Could you check a few things on this model? Use its own coordinates, in mm. Face numbers are marked on the shaded views. A direction names the side the tool comes from. Round coordinates to 2 decimals unless told otherwise and drop trailing zeros. Loops run counter-clockwise (first coordinate to the right, second up) from the corner with the lowest first, then second, coordinate; pieces in that order, holes last. Notation, with made-up numbers: M 66.25,39 L 73.25,39 A24 cw 73.25,70 Z; hole C 42,40.5 d2. An arc over 180 degrees is marked long. One line per item, written item: value. Start each with the question number.
Q1. Imagine slicing it at B-B (y = -62). Please give me the cut outline in (x, z).
Q2. Imagine slicing it at C-C (z = 29.95). Give the number of separate pieces and of enclosed holes in the cut face, then the cut area to 3 significant figures.
Q3. Which directions (+Z, -Z, +X, -X, +Y, -Y) give clear straight access to the entire face, cutting with the end or side of a thin tool? Please do the marked faces 4 and 5.
Q4. Imagine slicing it at A-A (z = 40). Please give me the cut outline in (x, y), then the cut area to 3 significant figures.
Q5. Thinking about a two-plate mould opening in Y: for the marked faces 1, 2 and 3, which applies, released by +Y, released by -Y, zero draft, split by the parting line, or undercut?
Q6. Please list where these lines run through material, in increasing order: line 1 along Y through (x, z) = (24.5, 20); line 2 along X through (y, z) = (-129, 64); line 3 along X through (y, z) = (7, 49.95).
Q7. Imagine slicing it at D-D (y = -124.5). Please give me the cut outline in (x, z), then the cut area to 3 significant figures.
Q8. I'm going to push flat-ended pins straight in: pin 1 Ø5.5 at (x, y) = (-38, -3) entering from -Z; pin 2 Ø10 at (x, y) = (19, -9.5) entering from +Z; pin 3 Ø9 at (x, y) = (-12, -93) entering from +Z. Where does each tip first touch, or does it pass through?
from build123d import *

# Parameters (mm, degrees)
SKETCH_1_W               = 160
SKETCH_1_H               = 170
EXTRUDE_1_DEPTH          = 3
SKETCH_9_W               = 160
SKETCH_9_H               = 170
SKETCH_9_W_2             = 154
SKETCH_9_H_2             = 164
EXTRUDE_6_DEPTH          = 75
SKETCH_10_R              = 4
SKETCH_10_R_2            = 1.55
EXTRUDE_7_DEPTH          = 20
SKETCH_11_W              = 14
SKETCH_11_H              = 14
CUT_EXTRUDE_3_DEPTH      = 20
SKETCH_12_R              = 22.5
CUT_EXTRUDE_4_DEPTH      = 10
SKETCH_13_W              = 15
SKETCH_13_H              = 35
CUT_EXTRUDE_5_DEPTH      = 10
SKETCH_14_W              = 10
SKETCH_14_H              = 10
EXTRUDE_8_DEPTH          = 10
SKETCH_15_W              = 4
SKETCH_15_H              = 7
CUT_EXTRUDE_6_DEPTH      = 10
SKETCH_16_R              = 1.6
CUT_EXTRUDE_7_DEPTH      = 20
MIRROR_4_COPY_1_SKETCH_W = 10
MIRROR_4_COPY_1_SKETCH_H = 10
MIRROR_4_COPY_1_DEPTH    = 10
MIRROR_4_COPY_2_SKETCH_W = 4
MIRROR_4_COPY_2_SKETCH_H = 7
MIRROR_4_COPY_2_DEPTH    = 10
MIRROR_4_COPY_3_SKETCH_R = 1.6
MIRROR_4_COPY_3_DEPTH    = 20
SKETCH_17_W              = 60
SKETCH_17_H              = 20
EXTRUDE_9_DEPTH          = 20
SKETCH_18_W              = 15
SKETCH_18_H              = 15
CUT_EXTRUDE_8_DEPTH      = 15
SKETCH_19_R              = 2.5
CUT_EXTRUDE_9_DEPTH      = 15
CUT_EXTRUDE_10_DEPTH     = 65


with BuildPart() as part:
    # 草图1 → 凸台-拉伸1 (new body)
    with BuildSketch(Plane.XY):
        with Locations((52.885281107, -76.271289123)):
            Rectangle(SKETCH_1_W, SKETCH_1_H)
    extrude(amount=EXTRUDE_1_DEPTH)

    # 草图9 → 凸台-拉伸6 (add)
    with BuildSketch(Plane.XY.offset(3)):
        with Locations((52.885281107, -76.271289123)):
            Rectangle(SKETCH_9_W, SKETCH_9_H)
        with Locations((52.885281107, -76.271289123)):
            Rectangle(SKETCH_9_W_2, SKETCH_9_H_2, mode=Mode.SUBTRACT)
    extrude(amount=EXTRUDE_6_DEPTH)

    # 草图10 → 凸台-拉伸7 (add)
    # profile 1 of 4: a face of its own
    with BuildSketch(Plane.XY.offset(3)):
        with Locations((-12.114718893, -0.271289123)):
            Circle(SKETCH_10_R)
        with Locations((-12.114718893, -0.271289123)):
            Circle(SKETCH_10_R_2, mode=Mode.SUBTRACT)
    # profile 2 of 4: a face of its own
    with BuildSketch(Plane.XY.offset(3)):
        with Locations((81.885281107, -0.271289123)):
            Circle(SKETCH_10_R)
        with Locations((81.885281107, -0.271289123)):
            Circle(SKETCH_10_R_2, mode=Mode.SUBTRACT)
    # profile 3 of 4: a face of its own
    with BuildSketch(Plane.XY.offset(3)):
        with Locations((-12.114718893, -94.271289123)):
            Circle(SKETCH_10_R)
        with Locations((-12.114718893, -94.271289123)):
            Circle(SKETCH_10_R_2, mode=Mode.SUBTRACT)
    # profile 4 of 4: a face of its own
    with BuildSketch(Plane.XY.offset(3)):
        with Locations((81.885281107, -94.271289123)):
            Circle(SKETCH_10_R)
        with Locations((81.885281107, -94.271289123)):
            Circle(SKETCH_10_R_2, mode=Mode.SUBTRACT)
    extrude(amount=EXTRUDE_7_DEPTH)

    # 草图11 → 切除-拉伸3 (cut)
    with BuildSketch(Plane(origin=(-24.114718893, 0, 0), x_dir=(0, 0, -1), z_dir=(1, 0, 0))):
        with Locations((-30.5, -83.221289123)):
            Rectangle(SKETCH_11_W, SKETCH_11_H)
    extrude(amount=-CUT_EXTRUDE_3_DEPTH, mode=Mode.SUBTRACT)

    # 草图12 → 切除-拉伸4 (cut)
    with BuildSketch(Plane.ZY.offset(27.114718893)):
        with Locations(Location((40, -126.271289123, 0), (0, 0, 270))):
            Circle(SKETCH_12_R)
    extrude(amount=-CUT_EXTRUDE_4_DEPTH, mode=Mode.SUBTRACT)

    # 草图13 → 切除-拉伸5 (cut)
    with BuildSketch(Plane.ZY.offset(27.114718893)):
        with Locations((55.5, -38.771289123)):
            Rectangle(SKETCH_13_W, SKETCH_13_H)
    extrude(amount=-CUT_EXTRUDE_5_DEPTH, mode=Mode.SUBTRACT)

    # 草图14 → 凸台-拉伸8 (add)
    with BuildSketch(Plane.XZ.offset(-5.728710877)):
        with Locations((-19.114718893, 73)):
            Rectangle(SKETCH_14_W, SKETCH_14_H)
    extrude_8 = extrude(amount=EXTRUDE_8_DEPTH)

    # 草图15 → 切除-拉伸6 (cut)
    with BuildSketch(Plane(origin=(-14.114718893, 0, 0), x_dir=(0, 0, -1), z_dir=(1, 0, 0))):
        with Locations((-72, 0.728710877)):
            Rectangle(SKETCH_15_W, SKETCH_15_H)
    cut_extrude_6 = extrude(amount=-CUT_EXTRUDE_6_DEPTH, mode=Mode.SUBTRACT)

    # 草图16 → 切除-拉伸7 (cut)
    with BuildSketch(Plane.XY.offset(78)):
        with Locations((-19.114718893, 0.728710877)):
            Circle(SKETCH_16_R)
    cut_extrude_7 = extrude(amount=-CUT_EXTRUDE_7_DEPTH, mode=Mode.SUBTRACT)

    # 镜向3: 凸台-拉伸8, 切除-拉伸6, 切除-拉伸7 across plane
    add(extrude_8.mirror(Plane.ZY.offset(-52.885281107)))
    add(cut_extrude_6.mirror(Plane.ZY.offset(-52.885281107)), mode=Mode.SUBTRACT)
    add(cut_extrude_7.mirror(Plane.ZY.offset(-52.885281107)), mode=Mode.SUBTRACT)

    # 镜向4: 凸台-拉伸8, 切除-拉伸6, 切除-拉伸7 across plane
    add(extrude_8.mirror(Plane.ZX.offset(-76.271289123)))
    add(cut_extrude_6.mirror(Plane.ZX.offset(-76.271289123)), mode=Mode.SUBTRACT)
    add(cut_extrude_7.mirror(Plane.ZX.offset(-76.271289123)), mode=Mode.SUBTRACT)

    # 镜向4 copy 1 sketch → 镜向4 copy 1 (add)
    with BuildSketch(Plane(origin=(105.770562214, -158.271289123, 0), x_dir=(-1, 0, 0), z_dir=(0, 1, 0))):
        with Locations((-19.114718893, 73)):
            Rectangle(MIRROR_4_COPY_1_SKETCH_W, MIRROR_4_COPY_1_SKETCH_H)
    extrude(amount=MIRROR_4_COPY_1_DEPTH)

    # 镜向4 copy 2 sketch → 镜向4 copy 2 (cut)
    with BuildSketch(Plane(origin=(119.885281107, -152.542578247, 0), x_dir=(0, 0, -1), z_dir=(-1, 0, 0))):
        with Locations((-72, 0.728710877)):
            Rectangle(MIRROR_4_COPY_2_SKETCH_W, MIRROR_4_COPY_2_SKETCH_H)
    extrude(amount=-MIRROR_4_COPY_2_DEPTH, mode=Mode.SUBTRACT)

    # 镜向4 copy 3 sketch → 镜向4 copy 3 (cut)
    with BuildSketch(Plane(origin=(105.770562214, -152.542578247, 78), x_dir=(-1, 0, 0), z_dir=(0, 0, 1))):
        with Locations((-19.114718893, 0.728710877)):
            Circle(MIRROR_4_COPY_3_SKETCH_R)
    extrude(amount=-MIRROR_4_COPY_3_DEPTH, mode=Mode.SUBTRACT)

    # 草图17 → 凸台-拉伸9 (add)
    with BuildSketch(Plane.ZY.offset(27.114718893)):
        with Locations((39, -1.271289123)):
            Rectangle(SKETCH_17_W, SKETCH_17_H)
    extrude_9 = extrude(amount=EXTRUDE_9_DEPTH)

    # 草图18 → 切除-拉伸8 (cut)
    with BuildSketch(Plane.ZY.offset(47.114718893)):
        with Locations((29.95, -3.771289123)):
            Rectangle(SKETCH_18_W, SKETCH_18_H)
        with Locations((49.95, -3.771289123)):
            Rectangle(SKETCH_18_W, SKETCH_18_H)
    cut_extrude_8 = extrude(amount=-CUT_EXTRUDE_8_DEPTH, mode=Mode.SUBTRACT)

    # 草图19 → 切除-拉伸9 (cut)
    with BuildSketch(Plane(origin=(0, 3.728710877, 0), x_dir=(-1, 0, 0), z_dir=(0, -1, 0))):
        with Locations(Location((39.614718893, -49.95, 0), (0, 0, 90))):
            Circle(SKETCH_19_R)
        with Locations(Location((39.614718893, -29.95, 0), (0, 0, 90))):
            Circle(SKETCH_19_R)
    cut_extrude_9 = extrude(amount=-CUT_EXTRUDE_9_DEPTH, mode=Mode.SUBTRACT)

    # 草图20 → 切除-拉伸10 (cut)
    with BuildSketch(Plane.XY.offset(69)):
        Polygon((-47.114718893, -11.271289123), (-27.114718893, -11.271289123), (-47.114718893, 5.558007734), align=None)
    cut_extrude_10 = extrude(amount=-CUT_EXTRUDE_10_DEPTH, mode=Mode.SUBTRACT)

    # 镜向5: 凸台-拉伸9, 切除-拉伸8, 切除-拉伸9, 切除-拉伸10 across plane
    add(extrude_9.mirror(Plane.ZY.offset(-52.885281107)))
    add(cut_extrude_8.mirror(Plane.ZY.offset(-52.885281107)), mode=Mode.SUBTRACT)
    add(cut_extrude_9.mirror(Plane.ZY.offset(-52.885281107)), mode=Mode.SUBTRACT)
    add(cut_extrude_10.mirror(Plane.ZY.offset(-52.885281107)), mode=Mode.SUBTRACT)


solid = part.part
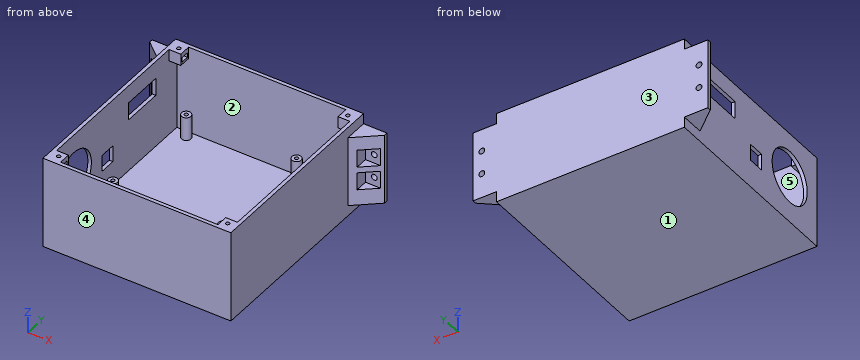
Report:
1. outline: M -27.11,0 L 132.89,0 L 132.89,78 L 129.89,78 L 129.89,3 L -24.11,3 L -24.11,78 L -27.11,78 Z
2. separate pieces: 4
2. enclosed holes: 0
2. area: 2,060 mm²
3. face 4: +Z, -Z, +X, -X, -Y
3. face 5: none
4. outline: M -47.11,5.56 L -27.11,-11.27 L -27.11,-103.77 L -24.11,-103.77 L -24.11,5.73 L 129.89,5.73 L 129.89,-158.27 L -24.11,-158.27 L -24.11,-148.77 L -27.11,-148.77 L -27.11,-161.27 L 132.89,-161.27 L 132.89,-11.27 L 152.89,5.56 L 152.89,8.73 L -47.11,8.73 Z
4. area: 2,270 mm²
5. face 1: zero draft
5. face 2: undercut
5. face 3: released by +Y
6. line 1: y = -161.27 to -158.27, 5.73 to 8.73
6. line 2: x = -27.11 to -24.11, 129.89 to 132.89
6. line 3: x = -47.11 to -42.11, -37.11 to 142.89, 147.89 to 152.89
7. outline: M -27.11,0 L 132.89,0 L 132.89,78 L 129.89,78 L 129.89,3 L -24.11,3 L -24.11,17.57 L -27.11,17.57 Z; M -27.11,62.43 L -24.11,62.43 L -24.11,78 L -27.11,78 Z
7. area: 795 mm²
8. pin 1: stops at z = 9
8. pin 2: stops at z = 3
8. pin 3: stops at z = 23
